Here's the drawing with two shaded views (mm, measured from the low corner). I have some questions. A direction names the side the tool comes from. Give positions to 0.01 mm unless a question says otherwise; leave off trailing zeros. Loops run counter-clockwise (first coordinate to the right, second up) from the corner with the lowest first, then second, coordinate; pieces in that order, holes last. Notation, with made-up numbers: (8.25, 39.5) - (43.25, 39.5) arc R22 ccw to (43.25, 61.5) - close; hole circle Ø9 at (-9.5, 20.5). An arc over 180 degrees is marked (long way). Write each question's results on one line, items separated by ' | '. Start each with the question number.
1) I want a section at B-B, the plane x = 2.25. Write out the boundary of the cut face in (y, z).
2) I want a section at C-C, the plane z = 1.5. Write out the boundary of the cut face in (x, y).
3) If I drill on probe 1 along X at (y, z) = (3.75, 3.25); probe 2 along Z at (x, y) = (0.5, 1.5); probe 3 along X at (y, z) = (0.75, 7), over which ranges is the centre line in solid material (lowest first)? Write a range as [from, to].
4) I'm going to push flat-ended pins straight in: pin 1 (0.8 mm diameter, centred on x = 0.5, z = 1.5, fed in from +Y); pin 2 (0.8 mm diameter, centred on x = 3.5, y = 2.5, fed in from -Z); pin 3 (0.5 mm diameter, centred on y = 5, z = 1.5, fed in from +X); pin 4 (2 mm diameter, centred on x = 1, z = 5.5, fed in from +Y). Where does each tip first touch, or does it pass through?
5) I want a section at A-A, the plane z = 3. Write out the boundary of the cut face in (x, y), and give its area (3 significant figures).
6) I want a section at D-D, the plane x = 1.5. Write out the boundary of the cut face in (y, z), and give its area (3 significant figures).
7) If we mould it in two halves opening along X, with no side actions, what happens to the marked faces 1, 2 and 3? For each: +X half, -X half, draft (parallel to the pull), parting line (faces both ways), or undercut.
8) On a 3-axis mill with a long thin cutter (end or side, diameter ignored), from which of +Z, -Z, +X, -X, +Y, -Y can I reach the whole of each face in a straight line? I mean the marked faces 4, 5, 6 and 7. Say none if no direction works.
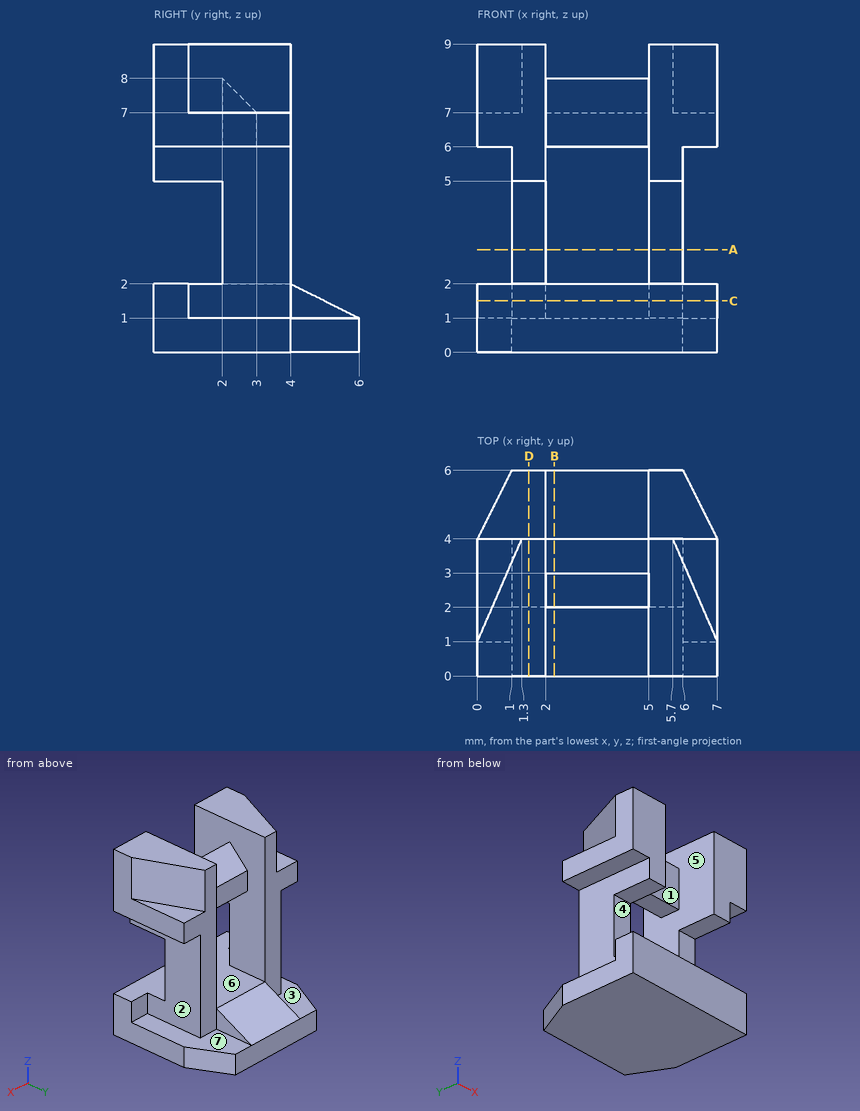
Answers:
1) outline: (0, 0) - (6, 0) - (6, 1) - (4, 2) - (0, 2) - close; (2, 6) - (3, 6) - (3, 7) - (2, 8) - close
2) outline: (0, 0) - (7, 0) - (7, 1) - (6, 1) - (6, 4) - (5, 4) - (5, 5) - (2, 5) - (2, 4) - (1, 4) - (1, 1) - (0, 1) - close
3) probe 1: x = [1, 2], [5, 6] | probe 2: z = [0, 1], [6, 9] | probe 3: x = [0, 2], [5, 7]
4) pin 1: stops at y = 1 | pin 2: stops at z = 0 | pin 3: stops at x = 5 | pin 4: stops at y = 4
5) outline: (1, 2) - (2, 2) - (2, 4) - (1, 4) - close; (5, 2) - (6, 2) - (6, 4) - (5, 4) - close | area: 4.00 mm2
6) outline: (0, 0) - (6, 0) - (6, 1) - (4, 1) - (4, 9) - (0, 9) - (0, 5) - (2, 5) - (2, 2) - (0, 2) - close | area: 32.0 mm2
7) face 1: undercut | face 2: +X half | face 3: draft
8) face 4: +X, -X, -Y | face 5: none | face 6: -Y | face 7: +X, +Y
